Here's how the part is built. I have some questions about the finished solid (model axes, mm). A direction names the side the tool comes from. Give positions to 0.01 mm unless a question says otherwise; leave off trailing zeros. Loops run counter-clockwise (first coordinate to the right, second up) from the corner with the lowest first, then second, coordinate; pieces in that order, holes last. Notation, with made-up numbers: M -32.75,81.25 L 21.25,81.25 A5 cw 21.25,88.25 Z; hole C -11,56.25 d11. An arc over 180 degrees is marked long. Write item = value, one per line. Start each with the question number.
```python
from build123d import *

# Parameters (mm, degrees)
SKETCH_1_W          = 100
SKETCH_1_H          = 130
EXTRUDE_1_DEPTH     = 3
SKETCH_2_W          = 20
SKETCH_2_H          = 25
EXTRUDE_2_DEPTH     = 37.25
FILLET_1_R          = 2
SKETCH_3_W          = 13
SKETCH_3_H          = 12
EXTRUDE_3_DEPTH     = 8
SKETCH_4_R          = 1.6
CUT_EXTRUDE_1_DEPTH = 95.135872546


with BuildPart() as part:
    # 草图1 → 凸台-拉伸1 (new body)
    with BuildSketch(Plane(origin=(0, 0, 0), x_dir=(1, 0, 0), z_dir=(0, 1, 0))):
        Rectangle(SKETCH_1_W, SKETCH_1_H)
    extrude(amount=EXTRUDE_1_DEPTH)

    # 草图2 → 凸台-拉伸2 (add)
    with BuildSketch(Plane(origin=(0, 3, 0), x_dir=(1, 0, 0), z_dir=(0, 1, 0))):
        with Locations((0, -52.5)):
            Rectangle(SKETCH_2_W, SKETCH_2_H)
        with Locations((25, -52.5)):
            Rectangle(SKETCH_2_W, SKETCH_2_H)
    extrude(amount=EXTRUDE_2_DEPTH)

    # 圆角1
    fillet_1_edges = [part.edges().sort_by_distance(p)[0] for p in [
        (-50, 1.5, 65),
        (-50, 1.5, -65),
        (50, 1.5, -65),
        (50, 1.5, 65),
    ]]
    fillet(fillet_1_edges, radius=FILLET_1_R)

    # 草图3 → 凸台-拉伸3 (add)
    with BuildSketch(Plane(origin=(0, 3, 0), x_dir=(1, 0, 0), z_dir=(0, 1, 0))):
        with Locations((50.5, 49)):
            Rectangle(SKETCH_3_W, SKETCH_3_H)
    extrude(amount=EXTRUDE_3_DEPTH)

    # 草图4 → 切除-拉伸1 (cut, through all)
    with BuildSketch(Plane(origin=(0, 3, 0), x_dir=(1, 0, 0), z_dir=(0, 1, 0))):
        with Locations(Location((-45, -60, 0), (0, 0, 270))):
            Circle(SKETCH_4_R)
        with Locations(Location((-45, 60, 0), (0, 0, 90))):
            Circle(SKETCH_4_R)
        with Locations(Location((45, 60, 0), (0, 0, 270))):
            Circle(SKETCH_4_R)
        with Locations(Location((45, -60, 0), (0, 0, 90))):
            Circle(SKETCH_4_R)
    extrude(amount=-CUT_EXTRUDE_1_DEPTH, mode=Mode.SUBTRACT)


solid = part.part
```
Q1. On a 3-axis mill with a long thin cutter (end or side, diameter ignored), from which of +Z, -Z, +X, -X, +Y, -Y can I reach the whole of each face in a straight line? I mean faces 1 (the flat face through (0, 21, 40)), 2 (the flat face through (15, 21, 53)), 3 (the flat face through (53, 3, -49)), 4 (the flat face through (35, 21, 53)). Say none if no direction works.
Q2. If I drill on line 1 along X through (y, z) = (1, -60); line 2 along X through (y, z) = (30.5, 42); line 3 along Y through (x, z) = (-45, 12.5), over which ranges is the centre line in solid material (lowest first)?
Q3. If we section it at A-A, the plane x = -45: List the corners of the cut face in (y, z) for me, then the cut area to 3 significant figures.
Q4. We'd pull the mould along Z, two halves only. Please class faces 5 (the cylindrical face through (-45.61, 1.52, 61.48)), 6 (the flat face through (-10, 21, 53)), 7 (the flat face through (50, 7, -43)): pulls with the +Z half, pulls with the -Z half, needs draft (parallel to the pull), parting line crosses it, or undercut.
Q5. Will these pins go through, and if not, where does the flat tip stop? pin 1 (2 mm diameter, centred on x = 5, z = 2.5, fed in from +Y); pin 2 (9 mm diameter, centred on x = 47.5, y = 8, fed in from +Z); pin 3 (4 mm diameter, centred on y = 5.5, z = -49.5, fed in from -X); pin 4 (3 mm diameter, centred on x = 45, z = -60, fed in from -Y).
Q6. If we section it at B-B, the plane z = 60: List the corners of the cut face in (x, y) for me, then the cut area to 3 significant figures.
Q7. If we section it at D-D, the plane z = -60: List the corners of the cut face in (x, y) for me.
Q8. If we section it at C-C, the plane y = 27: List the corners of the cut face in (x, z) for me.
Resolved:
q1.face_1 = -Z, +X, -X, +Y
q1.face_2 = +Z, -Z, +Y
q1.face_3 = +Z, -Z, +X, -Y
q1.face_4 = +Z, -Z, +X, +Y
q2.line_1 = -50 to -46.6, -43.4 to 43.4, 46.6 to 50
q2.line_2 = -10 to 10, 15 to 35
q2.line_3 = 0 to 3
q3.outline = M 0,-65 L 3,-65 L 3,-61.6 L 0,-61.6 Z; M 0,-58.4 L 3,-58.4 L 3,58.4 L 0,58.4 Z; M 0,61.6 L 3,61.6 L 3,65 L 0,65 Z
q3.area = 371 mm²
q4.face_5 = undercut
q4.face_6 = needs draft
q4.face_7 = pulls with the +Z half
q5.pin_1 = 3
q5.pin_2 = -43
q5.pin_3 = 44
q5.pin_4 = through
q6.outline = M -50,0 L -46.6,0 L -46.6,3 L -50,3 Z; M -43.4,0 L 43.4,0 L 43.4,3 L 35,3 L 35,40.25 L 15,40.25 L 15,3 L 10,3 L 10,40.25 L -10,40.25 L -10,3 L -43.4,3 Z; M 46.6,0 L 50,0 L 50,3 L 46.6,3 Z
q6.area = 1,770 mm²
q7.outline = M -50,0 L -46.6,0 L -46.6,3 L -50,3 Z; M -43.4,0 L 43.4,0 L 43.4,3 L -43.4,3 Z; M 46.6,0 L 50,0 L 50,3 L 46.6,3 Z
q8.outline = M -10,40 L 10,40 L 10,65 L -10,65 Z; M 15,40 L 35,40 L 35,65 L 15,65 Z
